Can you work these out from the model? Positions are in its coordinate system, mm. A direction names the side the tool comes from. Round coordinates to 2 decimals unless told otherwise and drop trailing zeros. Write each loop counter-clockwise with the first axis right and the second up, starting at its lowest first coordinate (ties: lowest second). Pieces come first, ordered by that corner, then holes. Notation, with made-up numbers: M -2.5,59 L 27.5,59 A8 cw 27.5,64 Z; hole C 84,24.25 d11. An arc over 180 degrees is marked long. Answer as a JSON object with one key per item and string values. Group by question number.
1) Suppose I cut it at C-C, the plane x = 61.5. Write out the boundary of the cut face in (y, z).
2) Suppose I cut it at B-B, the plane y = 189. Write out the boundary of the cut face in (x, z), and give its area (3 significant figures).
3) I'm going to push flat-ended pins straight in: pin 1 Ø8.5 at (x, y) = (-97.5, 232.5) entering from -Z; pin 2 Ø2 at (x, z) = (-24.5, -7.5) entering from -Y; pin 3 Ø2 at (x, y) = (99, 9) entering from +Z; pin 4 Ø11 at (y, z) = (29, -8) entering from +X. Where does each tip first touch, or does it pass through?
4) Please list where these lines run through material, in increasing order: L1, parallel to Y at x = 97.5, z = 9; L2, parallel to X at y = 7.5, z = 2.5; L3, parallel to Y at x = -97.5, z = 1.5. Write a range as [from, to].
5) On a 3-axis mill with a long thin cutter (end or side, diameter ignored), from which of +Z, -Z, +X, -X, +Y, -Y can I reach the whole of each face in a straight line? I mean faces 4 (the flat face through (0, 35, -10)), 5 (the cylindrical face through (-100.82, 232.94, 9.17)), 6 (the flat face through (-22.5, 30, -7)). Say none if no direction works.
6) If we mould it in two halves opening along Y, with no side actions, what happens to faces 1 (the flat face through (-1, 118, 10)), 2 (the flat face through (-1, 0, 5)), 3 (the flat face through (-42.5, 20, 5))? For each: +Y half, -Y half, draft (parallel to the pull), parting line (faces both ways), or undercut.
7) Suppose I cut it at A-A, the plane x = 15. Write out the boundary of the cut face in (y, z).
from build123d import *

# Parameters (mm, degrees)
SKETCH3_W           = 210
SKETCH3_H           = 10
BOSS_EXTRUDE1_DEPTH = 240
BOSS_EXTRUDE2_DEPTH = 205
SKETCH6_W           = 45
SKETCH6_H           = 15
BOSS_EXTRUDE3_DEPTH = 10
SKETCH7_R           = 1.65
CUT_EXTRUDE1_DEPTH  = 10
SKETCH8_W           = 21
SKETCH8_H           = 10
CUT_EXTRUDE2_DEPTH  = 10
SKETCH10_R          = 2.1
CUT_EXTRUDE3_DEPTH  = 4.5
FILLET2_R           = 5


with BuildPart() as part:
    # Sketch3 → Boss-Extrude1 (new body)
    with BuildSketch(Plane(origin=(0, 0, 0), x_dir=(1, 0, 0), z_dir=(0, 1, 0))):
        with Locations((0, -5)):
            Rectangle(SKETCH3_W, SKETCH3_H)
    extrude(amount=BOSS_EXTRUDE1_DEPTH)

    # Sketch5 → Boss-Extrude2 (add)
    with BuildSketch(Plane(origin=(0, 240, 0), x_dir=(1, 0, 0), z_dir=(0, 1, 0))):
        Polygon((-90, 0), (-90, 5), (90, 5), (90, 0), (105, 0), (105, -10), (-105, -10), (-105, 0), align=None)
    extrude(amount=-BOSS_EXTRUDE2_DEPTH)

    # Sketch6 → Boss-Extrude3 (add)
    with BuildSketch(Plane(origin=(0, 35, 0), x_dir=(1, 0, 0), z_dir=(0, 1, 0))):
        with Locations((0, 7.5)):
            Rectangle(SKETCH6_W, SKETCH6_H)
    extrude(amount=-BOSS_EXTRUDE3_DEPTH)

    # Sketch7 → Cut-Extrude1 (cut)
    with BuildSketch(Plane.XY.offset(10)):
        with Locations((-97.5, 232.5)):
            Circle(SKETCH7_R)
        with Locations((-97.5, 7.5)):
            Circle(SKETCH7_R)
        with Locations((97.5, 7.5)):
            Circle(SKETCH7_R)
        with Locations((97.5, 232.5)):
            Circle(SKETCH7_R)
    extrude(amount=-CUT_EXTRUDE1_DEPTH, mode=Mode.SUBTRACT)

    # Sketch8 → Cut-Extrude2 (cut)
    with BuildSketch(Plane.XY.offset(10)):
        with Locations((-32, 20)):
            Rectangle(SKETCH8_W, SKETCH8_H)
    extrude(amount=-CUT_EXTRUDE2_DEPTH, mode=Mode.SUBTRACT)

    # Sketch10 → Cut-Extrude3 (cut)
    with BuildSketch(Plane(origin=(0, 240, 0), x_dir=(1, 0, 0), z_dir=(0, 1, 0))):
        with Locations(Location((0, -2.5, 0), (0, 0, 270))):
            Circle(SKETCH10_R)
    extrude(amount=-CUT_EXTRUDE3_DEPTH, mode=Mode.SUBTRACT)

    # Sketch11 → CBORE for M3 SBHCS1 (revolve, cut)
    with BuildSketch(Plane(origin=(-97.5, 232.5, 10), x_dir=(0, -1, 0), z_dir=(1, 0, 0))):
        Polygon((0, 0), (0, 25), (1.7, 25), (1.7, 1.65), (3.35, 1.65), (3.35, 0.025), (3.375, 0), align=None)
    revolve(axis=Axis((-97.5, 232.5, 16.35), (0, 0, -1)), mode=Mode.SUBTRACT)

    # Sketch12 → CBORE for M3 SBHCS2 (revolve, cut)
    with BuildSketch(Plane(origin=(97.5, 232.5, 10), x_dir=(0, -1, 0), z_dir=(1, 0, 0))):
        Polygon((0, 0), (0, 25), (1.7, 25), (1.7, 1.65), (3.35, 1.65), (3.35, 0.025), (3.375, 0), align=None)
    revolve(axis=Axis((97.5, 232.5, 16.35), (0, 0, -1)), mode=Mode.SUBTRACT)

    # Sketch14 → CBORE for M3 SBHCS4 (revolve, cut)
    with BuildSketch(Plane(origin=(97.5, 7.5, 10), x_dir=(0, -1, 0), z_dir=(1, 0, 0))):
        Polygon((0, 0), (0, 25), (1.7, 25), (1.7, 1.65), (3.35, 1.65), (3.35, 0.025), (3.375, 0), align=None)
    revolve(axis=Axis((97.5, 7.5, 16.35), (0, 0, -1)), mode=Mode.SUBTRACT)

    # Sketch18 → CBORE for M3 SBHCS5 (revolve, cut)
    with BuildSketch(Plane(origin=(-97.5, 7.5, 10), x_dir=(0, -1, 0), z_dir=(1, 0, 0))):
        Polygon((0, 0), (0, 25), (1.7, 25), (1.7, 1.65), (3.35, 1.65), (3.35, 0.025), (3.375, 0), align=None)
    revolve(axis=Axis((-97.5, 7.5, 16.35), (0, 0, -1)), mode=Mode.SUBTRACT)

    # Fillet2
    # the kernel refuses this fillet: 5 mm, written as the material it takes off along each edge
    with BuildSketch(Plane(origin=(105, 252.5, 10), x_dir=(0, 0, -1), z_dir=(0, -1, 0)), Plane(origin=(-105, -12.5, 10), x_dir=(0, 0, -1), z_dir=(0, 1, 0))) as fillet2_piece_1:
        with BuildLine():
            CenterArc((FILLET2_R, -FILLET2_R), FILLET2_R, 90, 90)
            Line((0, -FILLET2_R), (0, 0))
            Line((0, 0), (FILLET2_R, 0))
        make_face()
    extrude(amount=265, mode=Mode.SUBTRACT)


solid = part.part
Results:
{
 "1": {"outline": "M 0,0 L 35,0 L 35,-5 L 240,-5 L 240,10 L 0,10 Z"},
 "2": {"outline": "M -105,0 L -90,0 L -90,-5 L 90,-5 L 90,0 L 105,0 L 105,5 A5 ccw 100,10 L -100,10 A5 ccw -105,5 Z", "area": "2,990 mm^2"},
 "3": {"pin 1": "z = 0", "pin 2": "through", "pin 3": "z = 8.35", "pin 4": "x = 22.5"},
 "4": {"L1": "[0, 4.15], [10.85, 229.15], [235.85, 240]", "L2": "[-105, -99.2], [-95.8, 95.8], [99.2, 105]", "L3": "[0, 5.8], [9.2, 230.8], [234.2, 240]"},
 "5": {"face 4": "-Z, +X, -X, +Y", "face 5": "+Z", "face 6": "-Z, -X, -Y"},
 "6": {"face 1": "draft", "face 2": "-Y half", "face 3": "undercut"},
 "7": {"outline": "M 0,0 L 25,0 L 25,-15 L 35,-15 L 35,-5 L 240,-5 L 240,10 L 0,10 Z"}
}
